Read the model definition and answer for the solid it produces. Units are mm, in the model's axes. Give positions to 0.01 mm unless a question says otherwise; leave off trailing zeros. Loops run counter-clockwise (first coordinate to the right, second up) from the corner with the lowest first, then second, coordinate; pieces in that order, holes last. Notation, with made-up numbers: (61.25, 74.5) - (71.25, 74.5) arc R26 ccw to (71.25, 108.5) - close; hole circle Ø8 at (-22, 32.5). An arc over 180 degrees is marked (long way). Write item = value, one per line. Start each with the question number.
Autodesk Inventor part; units mm, degrees
ref_plane "YZ Plane" through (0, 0, 0) normal (1, 0, 0) x (0, 1, 0)
ref_plane "XZ Plane" through (0, 0, 0) normal (0, 1, 0) x (-1, 0, 0)
ref_plane "XY Plane" through (0, 0, 0) normal (0, 0, 1) x (1, 0, 0)
sketch "スケッチ1" plane through (0, 0, 0) normal (0, 0, 1) x (1, 0, 0)
  circle A0 centre (2.8, 0) radius 2.8
  line L0 (2.8, 0) -> (0, 0)
  circle A1 centre (0, 2.8) radius 2.8
  circle A2 centre (-2.8, 0) radius 2.8
  circle A3 centre (0, -2.8) radius 2.8
  circle A4 centre (2.8, 0) radius 1.5
  circle A5 centre (0, 2.8) radius 1.5
  circle A6 centre (-2.8, 0) radius 1.5
  circle A7 centre (0, -2.8) radius 1.5
  circle A8 centre (0, 0) radius 5
  circle A9 centre (0, 5) radius 1.5
  circle A10 centre (-5, 0) radius 1.5
  circle A11 centre (0, -5) radius 1.5
  circle A12 centre (5, 0) radius 1.5
  point P0 (-1.483, -4.775)
  point P1 (1.483, -4.775)
  point P2 (-4.775, -1.483)
  point P3 (-4.775, 1.483)
  point P4 (4.775, 1.483)
  point P5 (4.775, -1.483)
  point P6 (-1.483, 4.775)
  point P7 (1.483, 4.775)
  dimension "d12" = 10
  dimension "d1" = 5.6
  dimension "d4" = 360
  dimension "d7" = 3
  dimension "d10" = 360
  dimension "d15" = 3
  dimension "d18" = 360
extrude "押し出し1" add sketch "スケッチ1" along normal blind 4 contours A8 A12 A4 A1 A0 | A0 A1 A8 | A8 A12 A4 | A8 A3 A0 | A0 A3 A4 A12 A8 | A1 A4 A0 A5 | A0 A5 A9 A8 A1 | A3 A8 A11 A7 A0 | A0 A7 A3 A4 | A9 A5 A8 | A8 A11 A7 | A0 A2 A5 | A4 L0 A1 | A9 A5 A2 A1 A8 | A7 A2 A0 | A3 L0 A4 | A8 A3 A2 A7 A11 | A3 A6 A1 | A1 A6 A2 A5 | A2 A7 A3 A6 | A1 A2 A8 | A8 A2 A3 | A1 A6 A10 A8 A2 | A2 A8 A10 A6 A3 | A10 A6 A8
extrude "押し出し2" add sketch "スケッチ1" along normal blind 1 contours A0 A12 A8 | A0 A12 | A9 A8 A1 | A1 A9 | A11 A3 | A3 A11 A8 | A10 A8 A2 | A2 A10 picked at (5.3837, -0.1736) picked at (-0.1045, 5.1773) picked at (-0.1045, -5.1773) picked at (-5.1773, 0.1045)
fillet "フィレット1" radius 1.05 8 edges at (4.775, 1.483, 0.5) (4.775, -1.483, 0.5) (1.483, 4.775, 0.5) (-1.483, 4.775, 0.5) (-1.483, -4.775, 0.5) (1.483, -4.775, 0.5) (-4.775, 1.483, 0.5) (-4.775, -1.483, 0.5)
properties part number "カムL4F" material "アセタール樹脂、白"
1. Consider line 1 along Y through (x, z) = (0, 1.8); line 2 along X through (y, z) = (0.75, 3.5). Determine where each line is inside the solid, lowest interval first. Write a range as [from, to].
2. For a pull along X with two mould halves and no side action, classify faces 1 (the flat face through (6, 0, 1)), 2 (the cylindrical face through (1.3, -0.07, 1.97)), 3 (the cylindrical face through (-5, 0, 2)), 4 (the cylindrical face through (-0.325, -1.336, 1.972)) as released by +X, released by -X, zero draft, split by the parting line, or undercut.
3. A cutting plane is placed at A-A on y = 0. Give the vertices of the cut face in (x, z).
4. Given P1, Ø1.6, axis at x = 0.5, y = -5.5, coming from the +Z side; P2, Ø1, axis at x = 1.5, z = 3, coming from the +Y side; P3, Ø1, axis at x = -6, y = 0.5, coming from the +Z side; P4, Ø1.5, axis at y = 4.5, z = 1.5, coming from the +X side, each flat-ended and moving along its own axis, determine where each tip first touches the part or whether it passes through.
5. A cutting plane is placed at C-C on z = 2.5. Give the vertices of the cut face in (x, y).
6. A cutting plane is placed at D-D on x = 3.25. Give the vertices of the cut face in (y, z).
Reply:
q1.line_1 = [-5, -4.3], [-1.3, 1.3], [4.3, 5]
q1.line_2 = [-4.94, -4.1], [-1.5, 1.5], [4.1, 4.94]
q2.face_1 = zero draft
q2.face_2 = undercut
q2.face_3 = split by the parting line
q2.face_4 = undercut
q3.outline = (-6.5, 0) - (-4.3, 0) - (-4.3, 4) - (-5, 4) - (-5, 1) - (-6.5, 1) - close; (-1.3, 0) - (1.3, 0) - (1.3, 4) - (-1.3, 4) - close; (4.3, 0) - (6.5, 0) - (6.5, 1) - (5, 1) - (5, 4) - (4.3, 4) - close
q4.P1 = 4
q4.P2 = 4.9
q4.P3 = 1
q4.P4 = 3.31
q5.outline = circle Ø10 at (0, 0); hole circle Ø3 at (-2.8, 0); hole circle Ø3 at (0, -2.8); hole circle Ø3 at (0, 2.8); hole circle Ø3 at (2.8, 0)
q6.outline = (-3.8, 0) - (-1.43, 0) - (-1.43, 4) - (-3.8, 4) - close; (1.43, 0) - (3.8, 0) - (3.8, 4) - (1.43, 4) - close
